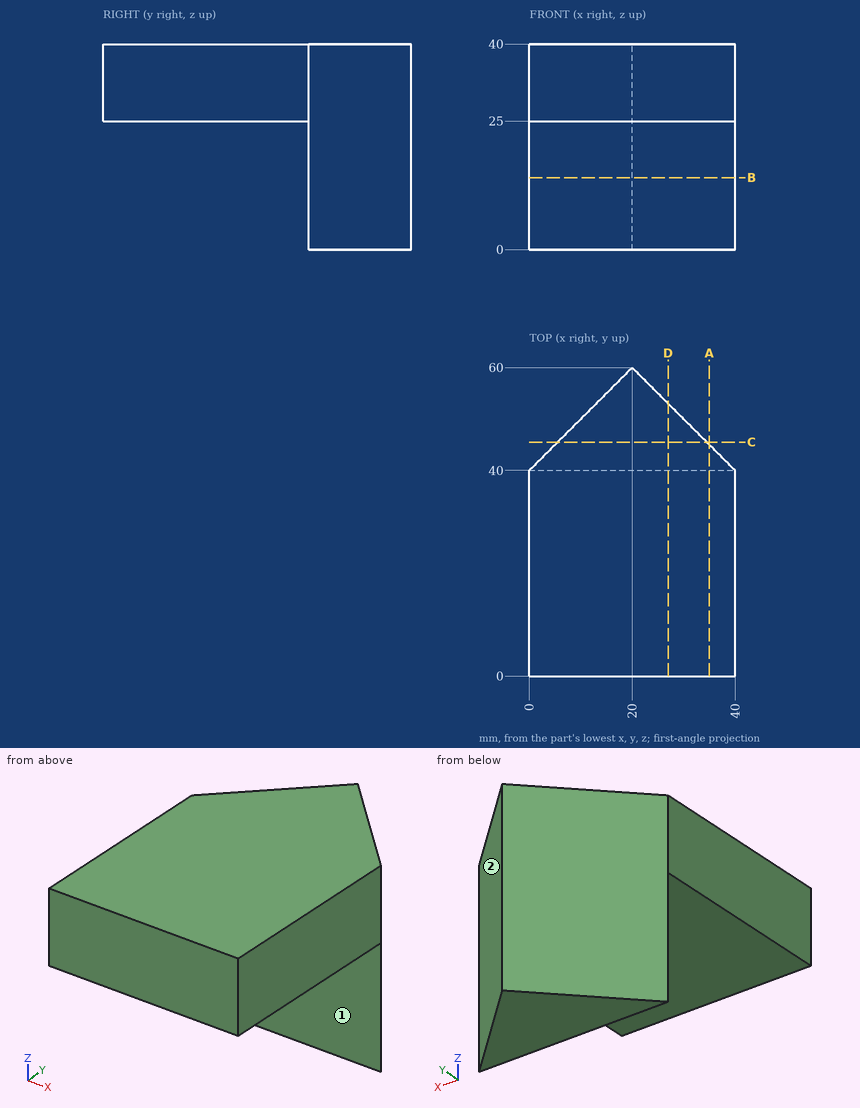
Part print with two shaded views. Sizes in mm from the minimum x, y, z corner. A direction names the side the tool comes from. Round coordinates to 2 decimals unless told otherwise and drop trailing zeros. Loops run counter-clockwise (first coordinate to the right, second up) from the corner with the lowest first, then second, coordinate; pieces in that order, holes last.
Item 1: Saw through at C-C (y = 45.5). List the corners of the cut face in (x, z), then the cut area to 3 significant figures.
Item 2: Drill centre lines: line 1 along Z through (x, y) = (18, 27.5); line 2 along Y through (x, z) = (8, 17.5); line 3 along X through (y, z) = (55, 36). Where is each one in solid material? Low to high.
Item 3: Saw through at B-B (z = 14). List the corners of the cut face in (x, y).
Item 4: Saw through at A-A (x = 35). List the corners of the cut face in (y, z), then the cut area to 3 significant figures.
Item 5: Pin check, flat tips, straight feed: P1, Ø4, axis at y = 43, z = 18.5, coming from the +X side; P2, Ø1, axis at x = 8, z = 27.5, coming from the +Y side; P3, Ø12, axis at x = 16, y = 15.5, coming from the -Z side. Stop position of each tip, or through.
Item 6: Saw through at D-D (x = 27). List the corners of the cut face in (y, z).
Item 7: Which spindle directions (+Z, -Z, +X, -X, +Y, -Y) get a long thin tool onto all of the face, cutting with end or side? Do the marked faces 1 and 2. Say none if no direction does.
Worked answers:
1. outline: (5.5, 0) - (34.5, 0) - (34.5, 40) - (5.5, 40) - close
1. area: 1,160 mm2
2. line 1: z = 25 to 40
2. line 2: y = 40 to 48
2. line 3: x = 15 to 25
3. outline: (0, 40) - (40, 40) - (20, 60) - close
4. outline: (0, 25) - (40, 25) - (40, 0) - (45, 0) - (45, 40) - (0, 40) - close
4. area: 800 mm2
5. P1: stops at x = 39
5. P2: stops at y = 48.5
5. P3: stops at z = 25
6. outline: (0, 25) - (40, 25) - (40, 0) - (53, 0) - (53, 40) - (0, 40) - close
7. face 1: -Z, +X, -X, -Y
7. face 2: +Z, -Z, +X, +Y
